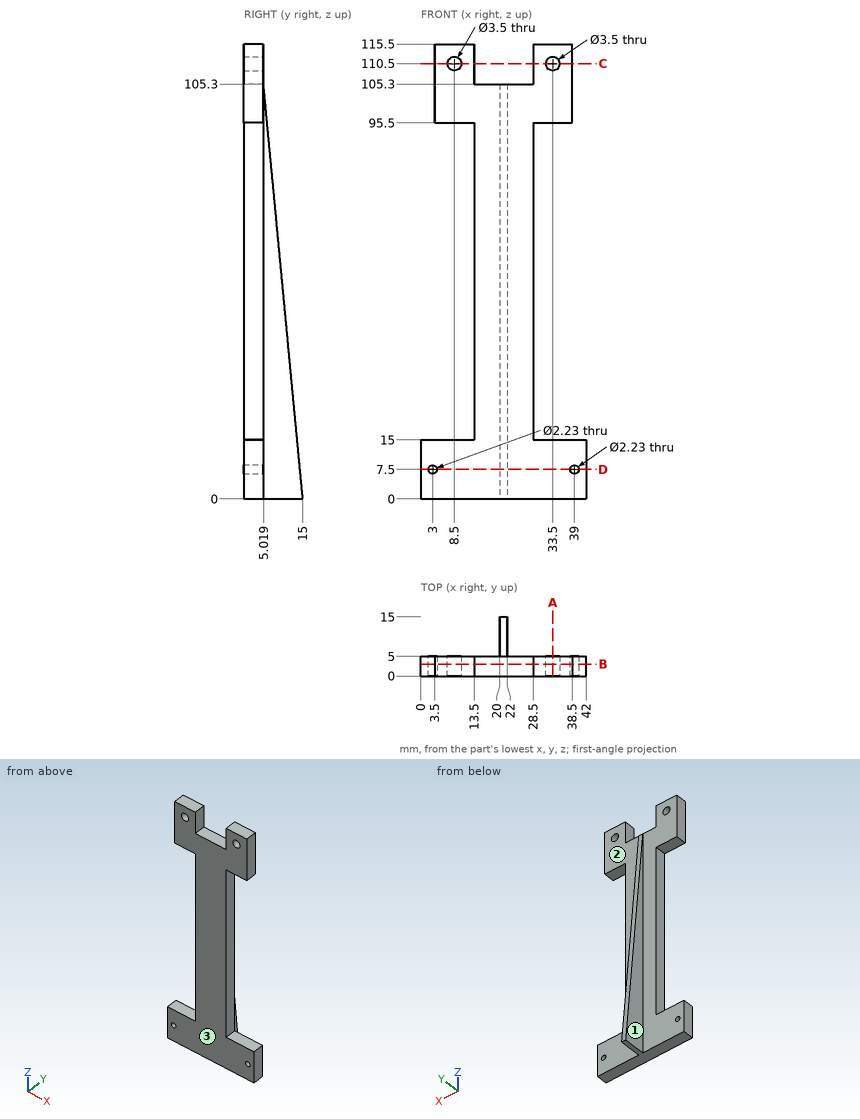
Source: three-view drawing plus pictorial views. Frame: mm from the lowest corner of the part. A direction names the side the tool comes from. Coordinates: 2 decimals unless noted, no trailing zeros. Loops run counter-clockwise (first coordinate to the right, second up) from the corner with the lowest first, then second, coordinate; pieces in that order, holes last. Notation, with made-up numbers: (1.25, -16) - (46.25, -16) arc R24 cw to (46.25, 14) - close; hole circle Ø5 at (-35, 28.25). An arc over 180 degrees is marked (long way). One line per item, written item: value. Start each with the question number.
1. Section A-A (x = 33.5). Return the cut outline in (y, z).
2. Set-up query: the marked faces 1, 2 and 3. Return all of +Z, -Z, +X, -X, +Y, -Y with unobstructed straight access to the full face (end or side cutting, diameter ignored); none if empty.
3. Section C-C (z = 110.5). Return the cut outline in (x, y).
4. Section D-D (z = 7.5). Return the cut outline in (x, y) (3 decimals).
5. Section B-B (y = 3). Return the cut outline in (x, z) (3 decimals).
6. Contact query for flat-ended pins moving along their axis: P1, Ø1.5, axis at y = 2.5, z = 109, coming from the -X side; P2, Ø2.5, axis at y = 3, z = 47, coming from the +X side; P3, Ø8, axis at y = 9.5, z = 47, coming from the -X side. Output: stop coordinate, or through.
7. Ray query, L1, parallel to Z at x = 33.5, y = 1.05; L2, parallel to X at y = 2.7, z = 110.5; L3, parallel to Z at x = 3, y = 1.1 (3 decimals). Return the intervals inside material, ascending.
Verdict:
1. outline: (0, 0) - (5, 0) - (5, 15) - (0, 15) - close; (0, 95.5) - (5, 95.5) - (5, 108.75) - (0, 108.75) - close; (0, 112.25) - (5, 112.25) - (5, 115.5) - (0, 115.5) - close
2. face 1: +Z, -Z, -X, +Y
2. face 2: +Z, -Z, +X, +Y
2. face 3: +Z, -Z, +X, -X, -Y
3. outline: (3.5, 0) - (6.75, 0) - (6.75, 5) - (3.5, 5) - close; (10.25, 0) - (13.5, 0) - (13.5, 5) - (10.25, 5) - close; (28.5, 0) - (31.75, 0) - (31.75, 5) - (28.5, 5) - close; (35.25, 0) - (38.5, 0) - (38.5, 5) - (35.25, 5) - close
4. outline: (0, 0) - (1.885, 0) - (1.885, 5) - (0, 5) - close; (4.115, 0) - (37.885, 0) - (37.885, 5) - (22, 5) - (22, 14.289) - (20, 14.289) - (20, 5) - (4.115, 5) - close; (40.115, 0) - (42, 0) - (42, 5) - (40.115, 5) - close
5. outline: (0, 0) - (42, 0) - (42, 15) - (28.5, 15) - (28.5, 95.5) - (38.5, 95.5) - (38.5, 115.5) - (28.5, 115.5) - (28.5, 105.3) - (13.5, 105.3) - (13.5, 115.5) - (3.5, 115.5) - (3.5, 95.5) - (13.5, 95.5) - (13.5, 15) - (0, 15) - close; hole circle Ø2.23 at (3, 7.5); hole circle Ø3.5 at (8.5, 110.5); hole circle Ø3.5 at (33.5, 110.5); hole circle Ø2.23 at (39, 7.5)
6. P1: stops at x = 3.5
6. P2: stops at x = 28.5
6. P3: stops at x = 20
7. L1: z = 0 to 15, 95.5 to 108.75, 112.25 to 115.5
7. L2: x = 3.5 to 6.75, 10.25 to 13.5, 28.5 to 31.75, 35.25 to 38.5
7. L3: z = 0 to 6.385, 8.615 to 15
